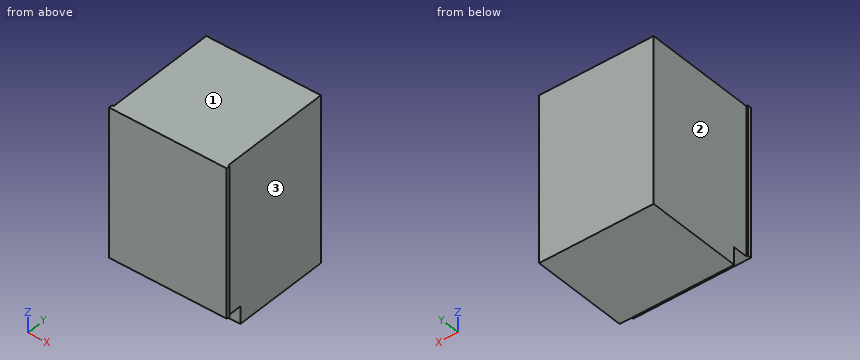
from build123d import *

# Parameters (mm, degrees)
F0_W     = 594
F0_H     = 860
F1_DEPTH = 600
F2_W     = 8
F2_H     = 860
F3_DEPTH = 19
F4_W     = 610
F4_H     = 90
F5_DEPTH = 95


with BuildPart() as f1:
    # F0 (on Front) → F1 (new body)
    with BuildSketch(Plane.XZ):
        with Locations((297, 430)):
            Rectangle(F0_W, F0_H)
    extrude(amount=F1_DEPTH)

    # F2 (on face) → F3 (join)
    with BuildSketch(Plane.XZ.offset(600)):
        with Locations((-4, 430)):
            Rectangle(F2_W, F2_H)
        with Locations((598, 430)):
            Rectangle(F2_W, F2_H)
    extrude(amount=-F3_DEPTH)

    # F4 (on face) → F5 (cut)
    with BuildSketch(Plane.XZ.offset(600)):
        with Locations((297, 45)):
            Rectangle(F4_W, F4_H)
    extrude(amount=-F5_DEPTH, mode=Mode.SUBTRACT)


solid = f1.part
Here's how the part is built. I have some questions about the finished solid (model axes, mm). Face numbers are marked on the shaded views. A direction names the side the tool comes from. Coordinates: 2 decimals unless noted, no trailing zeros. Loops run counter-clockwise (first coordinate to the right, second up) from the corner with the lowest first, then second, coordinate; pieces in that order, holes last. Notation, with made-up numbers: (27.5, 65) -> (34.5, 65) arc R14 cw to (34.5, 73) -> close; hole circle Ø2 at (-8, 87.5). An arc over 180 degrees is marked (long way). Use one line per item in the form item = value. Start each with the question number.
(1) If we section it at C-C (y = -262): Please give me the cut outline in (x, z).
(2) If we section it at A-A (z = 337.5): Please give me the cut outline in (x, y), then the cut area to 3 significant figures.
(3) On a 3-axis mill with a long thin cutter (end or side, diameter ignored), from which of +Z, -Z, +X, -X, +Y, -Y can I reach the whole of each face in a straight line? I mean the marked faces 1, 2 and 3. Say none if no direction works.
(4) If we section it at D-D (y = -521.5): Please give me the cut outline in (x, z).
(5) If we section it at B-B (x = 225): Please give me the cut outline in (y, z), then the cut area to 3 significant figures.
(6) Will these pins go through, and if not, where does the flat tip stop? pin 1 (10 mm diameter, centred on y = -342, z = 330.5, fed in from +X); pin 2 (1.5 mm diameter, centred on y = -483, z = 93.5, fed in from -X); pin 3 (4 mm diameter, centred on x = -2.5, z = 661, fed in from +Y).
(7) Please list where these lines run through material, in increasing order: line 1 along Y through (x, z) = (329, 54.5); line 2 along X through (y, z) = (-204.5, 131); line 3 along Z through (x, y) = (49, -568).
Verdict:
q1.outline = (0, 0) -> (594, 0) -> (594, 860) -> (0, 860) -> close
q2.outline = (-8, -600) -> (602, -600) -> (602, -581) -> (594, -581) -> (594, 0) -> (0, 0) -> (0, -581) -> (-8, -581) -> close
q2.area = 357,000 mm²
q3.face_1 = +Z, +X, -X, +Y, -Y
q3.face_2 = +Z, -Z, -X, +Y
q3.face_3 = +Z, -Z, +X, +Y
q4.outline = (0, 90) -> (594, 90) -> (594, 860) -> (0, 860) -> close
q5.outline = (-600, 90) -> (-505, 90) -> (-505, 0) -> (0, 0) -> (0, 860) -> (-600, 860) -> close
q5.area = 507,000 mm²
q6.pin_1 = 594
q6.pin_2 = 0
q6.pin_3 = -581
q7.line_1 = -505 to 0
q7.line_2 = 0 to 594
q7.line_3 = 90 to 860
